Autodesk Fusion 360 part; units mm, degrees
sketch "Sketch1" plane through (0, 0, 0) normal (0, 0, 1) x (1, 0, 0)
  line L0 (0, 0) -> (53.2, 0)
  line L1 (53.2, 0) -> (53.2, 40.2)
  line L2 (53.2, 40.2) -> (0, 40.2)
  line L3 (0, 40.2) -> (0, 0)
  circle A0 centre (4.6, 35.6) radius 1.6
  circle A1 centre (4.6, 4.6) radius 1.6
  circle A2 centre (48.6, 35.6) radius 1.6
  circle A3 centre (48.6, 4.6) radius 1.6
  dimension "d1" = 53.2
  dimension "d2" = 40.2
  dimension "d3" = 3.2
  dimension "d4" = 3.2
  dimension "d5" = 3.2
  dimension "d6" = 3.2
  dimension "d7" = 4.6
  dimension "d8" = 4.6
  dimension "d9" = 4.6
  dimension "d10" = 4.6
  dimension "d11" = 4.6
  dimension "d12" = 4.6
  dimension "d13" = 4.6
  dimension "d14" = 4.6
extrude "Extrude1" add sketch "Sketch1" along normal blind 4
sketch "Sketch2" plane through (0, 0, 0) normal (0, 0, -1) x (-1, 0, 0)
  circle A0 centre (-48.6, 4.6) radius 1.6
  circle A1 centre (-4.6, 4.6) radius 1.6
  circle A2 centre (-48.6, 35.6) radius 1.6
  circle A3 centre (-4.6, 35.6) radius 1.6
  line L0 (0, 0) -> (0, 40.2)
  line L1 (0, 40.2) -> (-53.2, 40.2)
  line L2 (-53.2, 40.2) -> (-53.2, 0)
  line L3 (-53.2, 0) -> (0, 0)
  line L4 (-3.0123, 32.85) -> (-1.4246, 35.6)
  line L5 (-1.4246, 35.6) -> (-3.0123, 38.35)
  line L6 (-3.0123, 38.35) -> (-6.1877, 38.35)
  line L7 (-6.1877, 38.35) -> (-7.7754, 35.6)
  line L8 (-7.7754, 35.6) -> (-6.1877, 32.85)
  line L9 (-6.1877, 32.85) -> (-3.0123, 32.85)
  line L10 (-47.0123, 32.85) -> (-45.4246, 35.6)
  line L11 (-45.4246, 35.6) -> (-47.0123, 38.35)
  line L12 (-47.0123, 38.35) -> (-50.1877, 38.35)
  line L13 (-50.1877, 38.35) -> (-51.7754, 35.6)
  line L14 (-51.7754, 35.6) -> (-50.1877, 32.85)
  line L15 (-50.1877, 32.85) -> (-47.0123, 32.85)
  line L16 (-50.1877, 7.35) -> (-51.7754, 4.6)
  line L17 (-51.7754, 4.6) -> (-50.1877, 1.85)
  line L18 (-50.1877, 1.85) -> (-47.0123, 1.85)
  line L19 (-47.0123, 1.85) -> (-45.4246, 4.6)
  line L20 (-45.4246, 4.6) -> (-47.0123, 7.35)
  line L21 (-47.0123, 7.35) -> (-50.1877, 7.35)
  line L22 (-6.1877, 7.35) -> (-7.7754, 4.6)
  line L23 (-7.7754, 4.6) -> (-6.1877, 1.85)
  line L24 (-6.1877, 1.85) -> (-3.0123, 1.85)
  line L25 (-3.0123, 1.85) -> (-1.4246, 4.6)
  line L26 (-1.4246, 4.6) -> (-3.0123, 7.35)
  line L27 (-3.0123, 7.35) -> (-6.1877, 7.35)
  dimension "d17" = 2.75
  dimension "d18" = 2.75
  dimension "d19" = 2.75
  dimension "d20" = 2.75
extrude "Extrude2" cut sketch "Sketch2" against normal blind 2 contours L4 L5 L6 L7 L8 L9 | L10 L11 L12 L13 L14 L15 | L16 L17 L18 L19 L20 L21 | L22 L23 L24 L25 L26 L27
fillet "Fillet1" radius 4.6 4 edges at (53.2, 40.2, 2) (53.2, 0, 2) (0, 0, 2) (0, 40.2, 2)
sketch "Sketch4" plane through (0, 0, 4) normal (0, 0, 1) x (1, 0, 0)
  arc A0 (4.6, 40.2) -> (0, 35.6) centre (4.6, 35.6) ccw
  line L0 (0, 35.6) -> (0, 4.6)
  arc A1 (0, 4.6) -> (4.6, 0) centre (4.6, 4.6) ccw
  line L1 (4.6, 0) -> (48.6, 0)
  arc A2 (48.6, 0) -> (53.2, 4.6) centre (48.6, 4.6) ccw
  line L2 (53.2, 4.6) -> (53.2, 35.6)
  arc A3 (53.2, 35.6) -> (48.6, 40.2) centre (48.6, 35.6) ccw
  line L3 (48.6, 40.2) -> (4.6, 40.2)
  circle A4 centre (4.6, 4.6) radius 1.6
  circle A5 centre (48.6, 35.6) radius 1.6
  circle A6 centre (4.6, 35.6) radius 1.6
  circle A7 centre (48.6, 4.6) radius 1.6
  line L4 (1.2, 35.6) -> (1.2, 4.6)
  arc A8 (1.2, 4.6) -> (4.6, 1.2) centre (4.6, 4.6) ccw
  line L5 (4.6, 1.2) -> (48.6, 1.2)
  arc A9 (48.6, 1.2) -> (52, 4.6) centre (48.6, 4.6) ccw
  line L6 (52, 4.6) -> (52, 35.6)
  arc A10 (52, 35.6) -> (48.6, 39) centre (48.6, 35.6) ccw
  line L7 (48.6, 39) -> (4.6, 39)
  arc A11 (4.6, 39) -> (1.2, 35.6) centre (4.6, 35.6) ccw
  dimension "d24" = 1.2
extrude "Extrude3" add sketch "Sketch4" along normal blind 1.6 contours A0 L0 A1 L1 A2 L2 A3 L3
sketch "Sketch5" plane through (0, 0, 4) normal (0, 0, 1) x (1, 0, 0)
  line L0 (1.2, 35.6) -> (1.2, 4.6)
  arc A0 (1.2, 4.6) -> (4.6, 1.2) centre (4.6, 4.6) ccw
  line L1 (4.6, 1.2) -> (48.6, 1.2)
  arc A1 (48.6, 1.2) -> (52, 4.6) centre (48.6, 4.6) ccw
  line L2 (52, 4.6) -> (52, 35.6)
  arc A2 (52, 35.6) -> (48.6, 39) centre (48.6, 35.6) ccw
  line L3 (48.6, 39) -> (4.6, 39)
  arc A3 (4.6, 39) -> (1.2, 35.6) centre (4.6, 35.6) ccw
  circle A4 centre (4.6, 4.6) radius 1.6
  circle A5 centre (48.6, 35.6) radius 1.6
  circle A6 centre (4.6, 35.6) radius 1.6
  circle A7 centre (48.6, 4.6) radius 1.6
  line L4 (1.2, 13.2) -> (6.6, 13.2)
  line L5 (6.6, 13.2) -> (6.6, 1.2)
  line L6 (46.6, 1.2) -> (46.6, 6.6)
  line L7 (46.6, 6.6) -> (52, 6.6)
  line L8 (1.2, 27) -> (6.6, 27)
  line L9 (6.6, 27) -> (6.6, 39)
  line L10 (46.6, 39) -> (46.6, 33.6)
  line L11 (46.6, 33.6) -> (52, 33.6)
  dimension "d27" = 12
  dimension "d28" = 5.4
  dimension "d29" = 5.4
  dimension "d30" = 12
  dimension "d31" = 5.4
  dimension "d32" = 5.4
  dimension "d33" = 5.4
  dimension "d34" = 5.4
extrude "Extrude4" cut sketch "Sketch5" against normal blind 1.5 contours L0 L1 L2 L3 L4 L5 L6 L7 L8 L9 L10 L11
sketch "Sketch6" plane through (0, 0, 5.6) normal (0, 0, 1) x (1, 0, 0)
  arc A0 (4.6, 39) -> (1.2, 35.6) centre (4.6, 35.6) ccw
  line L0 (4.6, 39) -> (48.6, 39)
  arc A1 (52, 35.6) -> (48.6, 39) centre (48.6, 35.6) ccw
  line L1 (52, 35.6) -> (52, 4.6)
  arc A2 (48.6, 1.2) -> (52, 4.6) centre (48.6, 4.6) ccw
  line L2 (48.6, 1.2) -> (4.6, 1.2)
  arc A3 (1.2, 4.6) -> (4.6, 1.2) centre (4.6, 4.6) ccw
  line L3 (1.2, 4.6) -> (1.2, 35.6)
  line L4 (48.6, 40.2) -> (4.6, 40.2)
  arc A4 (4.6, 40.2) -> (0, 35.6) centre (4.6, 35.6) ccw
  line L5 (0, 35.6) -> (0, 4.6)
  arc A5 (0, 4.6) -> (4.6, 0) centre (4.6, 4.6) ccw
  line L6 (4.6, 0) -> (48.6, 0)
  arc A6 (48.6, 0) -> (53.2, 4.6) centre (48.6, 4.6) ccw
  line L7 (53.2, 4.6) -> (53.2, 35.6)
  arc A7 (53.2, 35.6) -> (48.6, 40.2) centre (48.6, 35.6) ccw
  line L8 (0, 25.1) -> (1.2, 25.1)
  line L9 (0, 15.1) -> (1.2, 15.1)
  dimension "d37" = 10
  dimension "d38" = 10.5
extrude "Extrude5" cut sketch "Sketch6" against normal blind 1.6 contours L3 L5 L8 L9
fillet "Fillet2" radius 1.6 2 edges at (0.6, 25.1, 4) (0.6, 15.1, 4)
equation "d1 = 50 mm + ( ( 2 * 1.6 ) * 1 mm )"
equation "d2 = 37 mm + ( ( 2 * 1.6 ) * 1 mm )"
equation "d7 = 3 mm + 1.6 mm"
equation "d8 = d7"
equation "d9 = d7"
equation "d10 = d7"
equation "d11 = d7"
equation "d12 = d7"
equation "d13 = d7"
equation "d14 = d7"
equation "d17 = ( 5.5 / 2 ) * 1 mm"
equation "d18 = d17"
equation "d19 = d17"
equation "d20 = d17"
equation "d23 = 3 mm + 1.6 mm"
equation "d28 = 5 mm + 0.4 mm"
equation "d29 = d28"
equation "d30 = d27"
equation "d31 = d34"
equation "d32 = d28"
equation "d33 = d32"
Geometry check sheet. Reference: the model listing, model coordinates, mm. A direction names the side the tool comes from. Give positions to 0.01 mm unless a question says otherwise; leave off trailing zeros. Order: outer loops, then holes, each group sorted by start corner. A loop starts at its lowest first (then second) coordinate and runs counter-clockwise, first axis right, second up.
1. Section check B-B, the plane y = 21. Enter the section's corners in (x, z).
2. Gauge pin test, flat ends, axial feed: pin 1 Ø3.5 at (x, y) = (4.6, 4.6) entering from +Z; pin 2 Ø1.9 at (x, y) = (4.6, 35.6) entering from +Z; pin 3 Ø10 at (x, y) = (18.5, 19.5) entering from +Z. Record the tip position at first contact, or that the pin passes through.
3. Access from +Z, -Z, +X, -X, +Y, -Y to the whole of each face (thin tool, end or side, straight path). Record for faces 1 (the face through (4, 32, 4)), 2 (the face through (5, 7.35, 1)).
4. Thickness scan on L1, parallel to Y at x = 48.6, z = 3.65; L2, parallel to Y at x = 4.6, z = 2.9; L3, parallel to Y at x = 4.6, z = 2.45. Record the ranges inside material, lowest first.
5. Section check C-C, the plane x = 30. Enter the section's corners in (y, z), and give its area (3 significant figures).
6. Release check for a two-part mould opening along X. For faces 3 (the face through (27, 40.2, 3)), 4 (the face through (53.2, 20, 3)), 5 (the face through (50.98, 38.03, 4.79)) record: pulls with the +X half, pulls with the -X half, needs draft (parallel to the pull), parting line crosses it, or undercut.
7. Section check A-A, the plane z = 1.2. Give the number of separate pieces and of enclosed holes in the cut face, and give its area (3 significant figures).
Values follow:
1. outline: (0, 0) - (53.2, 0) - (53.2, 5.6) - (52, 5.6) - (52, 2.5) - (1.2, 2.5) - (1.2, 4) - (0, 4) - close
2. pin 1: stops at z = 4
2. pin 2: passes through
2. pin 3: stops at z = 2.5
3. face 1: +Z
3. face 2: -Z
4. L1: y = 0 to 3, 6.2 to 6.6, 33.6 to 34, 37.2 to 40.2
4. L2: y = 0 to 3, 6.2 to 13.2, 27 to 34, 37.2 to 40.2
4. L3: y = 0 to 3, 6.2 to 34, 37.2 to 40.2
5. outline: (0, 0) - (40.2, 0) - (40.2, 5.6) - (39, 5.6) - (39, 2.5) - (1.2, 2.5) - (1.2, 5.6) - (0, 5.6) - close
5. area: 108 mm2
6. face 3: needs draft
6. face 4: pulls with the +X half
6. face 5: undercut
7. separate pieces: 1
7. enclosed holes: 4
7. area: 2,020 mm2
